The listing builds one solid part. Answer for the finished solid, in the listing's coordinates (mm). Face numbers are marked on the shaded views. A direction names the side the tool comes from. Give positions to 0.01 mm unless a question says otherwise; leave off trailing zeros. Use a Markdown table: item, result. Add a question column.
1) The mould has two halves that part along Y. Classify the marked faces 1, 2 and 3: released by +Y, released by -Y, zero draft, split by the parting line, or undercut.
2) Flat-ended cylindrical pins translate along their axes: pin 1 (3 mm diameter, centred on x = 12, y = -58.5, fed in from +Z); pin 2 (6 mm diameter, centred on x = -6, y = 48.5, fed in from +Z); pin 3 (10 mm diameter, centred on x = 11.5, z = 6.5, fed in from -Y). Find the tip coordinate at first contact, or state that the pin passes through.
3) For the marked faces 4 and 5, determine the directions among +Z, -Z, +X, -X, +Y, -Y from which every point of the face is accessible in a straight line to the end or side of a thin tool.
4) Straight lines are drawn through the part: line 1 (Y direction, x = -1, z = 0); line 2 (Y direction, x = -6, z = -5.5); line 3 (X direction, y = 28, z = -24.5) (3 decimals). For each, find the intervals that lie inside material, in ascending order.
from build123d import *

# Parameters (mm, degrees)
CUT_EXTRUDE1_DEPTH      = 147.750959265
CUT_EXTRUDE1_DEPTH_BACK = 147.750959265


with BuildPart() as part:
    # Sketch1 → Revolve1 (revolve)
    with BuildSketch(Plane.XY, mode=Mode.PRIVATE) as revolve1_sk:
        with BuildLine():
            Line((-10.795, 0), (-10.795, 40.932303645))
            ThreePointArc((-10.795, 40.932303645), (-10.334179588, 44.322360135), (-8.985160157, 47.466399739))
            Line((-8.985160157, 47.466399739), (-4.984839843, 54.133600261))
            ThreePointArc((-4.984839843, 54.133600261), (-3.635820412, 57.277639865), (-3.175, 60.667696355))
            Line((-3.175, 60.667696355), (-3.175, 67.170867113))
            ThreePointArc((-3.175, 67.170867113), (-5.202068626, 74.054073915), (-10.636186753, 78.74))
            Line((-10.636186753, 78.74), (-19.05, 82.55))
            Line((-19.05, 82.55), (-19.05, 96.8375))
            ThreePointArc((-19.05, 96.8375), (-17.655096045, 100.205096045), (-14.2875, 101.6))
            Line((-14.2875, 101.6), (14.2875, 101.6))
            ThreePointArc((14.2875, 101.6), (17.655096045, 100.205096045), (19.05, 96.8375))
            Line((19.05, 96.8375), (19.05, 82.55))
            Line((19.05, 82.55), (10.636186753, 78.74))
            ThreePointArc((10.636186753, 78.74), (5.202068626, 74.054073915), (3.175, 67.170867113))
            Line((3.175, 67.170867113), (3.175, 60.667696355))
            ThreePointArc((3.175, 60.667696355), (3.635820412, 57.277639865), (4.984839843, 54.133600261))
            Line((4.984839843, 54.133600261), (8.985160157, 47.466399739))
            ThreePointArc((8.985160157, 47.466399739), (10.334179588, 44.322360135), (10.795, 40.932303645))
            Line((10.795, 40.932303645), (10.795, 0))
            Line((10.795, 0), (-10.795, 0))
        make_face()
    revolve(revolve1_sk.sketch.rotate(Axis((-10.795, 0, 0), (1, 0, 0)), 90), axis=Axis((-10.795, 0, 0), (1, 0, 0)))

    # Sketch2 → Cut-Extrude1 (cut, two sides: drawn at the far end of the back side and taken through both)
    with BuildSketch(Plane.ZY.offset(10.795).offset(-CUT_EXTRUDE1_DEPTH_BACK)):
        with BuildLine():
            Line((-7.079276607, -7.710444497), (-3.072643811, -10.301240032))
            Line((-3.072643811, -10.301240032), (-1.643427642, -7.765503965))
            ThreePointArc((-1.643427642, -7.765503965), (3.897381242, 6.914790359), (-5.792301857, -5.42707522))
            Line((-5.792301857, -5.42707522), (-7.079276607, -7.710444497))
        make_face()
    extrude(amount=CUT_EXTRUDE1_DEPTH + CUT_EXTRUDE1_DEPTH_BACK, mode=Mode.SUBTRACT)


solid = part.part
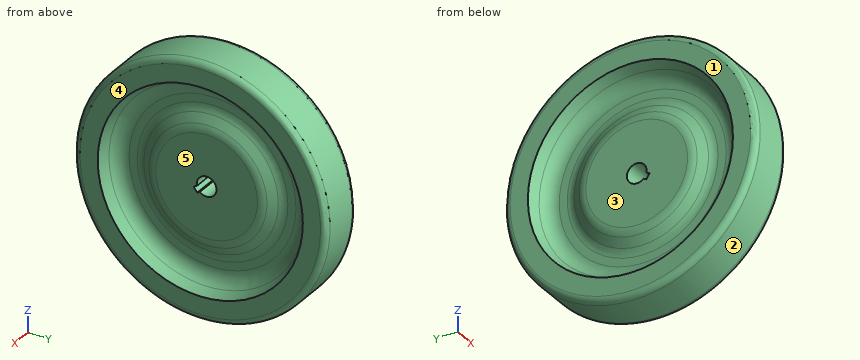
The answers:
| question | item | result |
|---|---|---|
| 1 | face 1 | zero draft |
| 1 | face 2 | split by the parting line |
| 1 | face 3 | undercut |
| 2 | pin 1 | z = 84.1 |
| 2 | pin 2 | z = 90.84 |
| 2 | pin 3 | y = -101.59 |
| 3 | face 4 | +Z, -Z, +X, +Y, -Y |
| 3 | face 5 | +X |
| 4 | line 1 | -101.6 to -7.94, 7.94 to 101.6 |
| 4 | line 2 | -101.45 to -74.96, -52.15 to -8.73, 5.72 to 52.15, 74.96 to 101.45 |
| 4 | line 3 | -10.795 to 10.795 |
